Check sheet for the modelled part. Datum: model origin and axes. Units: mm. Face numbers are marked on the shaded views. A direction names the side the tool comes from. Coordinates: 2 decimals unless noted, no trailing zeros. Write each loop counter-clockwise with the first axis right and the second up, starting at its lowest first coordinate (ties: lowest second). Pieces come first, ordered by that corner, then holes. Notation, with made-up numbers: (5, 30.25) -> (10, 30.25) arc R16 cw to (10, 50.25) -> close; hole circle Ø1 at (13, 85.5). An arc over 180 degrees is marked (long way). One line per item, written item: value. Start each with the question number.
1) Gauge pin test, flat ends, axial feed: P1, Ø4, axis at x = 3, z = -9, coming from the +Y side; P2, Ø1.5, axis at y = 4, z = -2, coming from the -X side; P3, Ø1.3, axis at x = -1, y = 4, coming from the +Z side; P4, Ø0.8, axis at x = 4.5, z = -14.5, coming from the +Y side. Record the tip position at first contact, or that the pin passes through.
2) Sectioned sample at C-C on y = 1.05. Give the number of separate pieces and of enclosed holes in the cut face, plus the area to 3 significant figures.
3) Sectioned sample at A-A on z = 0. Enter the section's corners in (x, y).
4) Sectioned sample at B-B on x = 15. Enter the section's corners in (y, z).
5) Set-up check for the marked faces 4, 5 and 6: record each of +Z, -Z, +X, -X, +Y, -Y from which the full face is reachable in a straight line by a thin tool's end or side.
6) Sectioned sample at D-D on z = -6. Enter the section's corners in (x, y), plus the area to 3 significant figures.
7) Draft check along X on the marked faces 1, 2 and 3. Enter one of: +X half, -X half, draft (parallel to the pull), parting line (faces both ways), or undercut.
8) Scan lines: line 1 along Z through (x, y) = (10, 3.4); line 2 along Y through (x, z) = (14.5, 7); line 3 along Z through (x, y) = (15.5, 0.3). Record each from-to range of solid material in increasing order. Write a range as [from, to].
```python
from build123d import *

# Parameters (mm, degrees)
SKETCH1_R           = 17.5
BOSS_EXTRUDE1_DEPTH = 0.5
SKETCH2_R           = 11.5
CUT_EXTRUDE1_DEPTH  = 0.5
SKETCH3_W           = 15
SKETCH3_H           = 8
CUT_EXTRUDE4_DEPTH  = 2.5
BOSS_EXTRUDE6_DEPTH = 4.5
BOSS_EXTRUDE7_START = 4
SKETCH9_R           = 12.2
SKETCH9_R_2         = 11.5
BOSS_EXTRUDE7_DEPTH = 4
SKETCH10_W          = 4.218070674
SKETCH10_H          = 8
CUT_EXTRUDE5_DEPTH  = 6
SKETCH11_R          = 1
SKETCH11_R_2        = 0.998714777
SKETCH11_R_3        = 0.998671431
SKETCH11_R_4        = 1.032567444
SKETCH11_R_5        = 1.008118798
CUT_EXTRUDE7_DEPTH  = 100


with BuildPart() as part:
    # Sketch1 → Boss-Extrude1 (new body)
    with BuildSketch(Plane(origin=(0, 0, 0), x_dir=(1, 0, 0), z_dir=(0, 1, 0))):
        with Locations(Location((0, 0, 0), (0, 0, 270))):
            Circle(SKETCH1_R)
    extrude(amount=BOSS_EXTRUDE1_DEPTH)

    # Sketch2 → Cut-Extrude1 (cut)
    with BuildSketch(Plane(origin=(0, 0.5, 0), x_dir=(1, 0, 0), z_dir=(0, 1, 0))):
        with Locations(Location((2, 0, 0), (0, 0, 270))):
            Circle(SKETCH2_R)
    extrude(amount=-CUT_EXTRUDE1_DEPTH, mode=Mode.SUBTRACT)

    # Sketch3 → Cut-Extrude4 (cut)
    with BuildSketch(Plane(origin=(0, 0, 0), x_dir=(1, 0, 0), z_dir=(0, 1, 0))):
        with Locations((-5.5, 0)):
            Rectangle(SKETCH3_W, SKETCH3_H)
    extrude(amount=CUT_EXTRUDE4_DEPTH, mode=Mode.SUBTRACT)

    # Sketch7 → Boss-Extrude6 (add)
    with BuildSketch(Plane(origin=(0, 0.5, 0), x_dir=(1, 0, 0), z_dir=(0, 1, 0))):
        with BuildLine():
            Line((-11.135528726, 13.5), (11.135528726, 13.5))
            ThreePointArc((11.135528726, 13.5), (10.820652744, 13.753671299), (10.5, 14))
            Line((10.5, 14), (-10.5, 14))
            ThreePointArc((-10.5, 14), (-10.820652744, 13.753671299), (-11.135528726, 13.5))
        make_face()
        with BuildLine():
            Line((12.176537068, 12.5), (-12.176537068, 12.5))
            ThreePointArc((-12.176537068, 12.5), (-12.42556977, 12.252480192), (-12.669572012, 12))
            Line((-12.669572012, 12), (12.669572012, 12))
            ThreePointArc((12.669572012, 12), (12.42556977, 12.252480192), (12.176537068, 12.5))
        make_face()
        with BuildLine():
            ThreePointArc((-11.145229996, -13.491992008), (-10.830835088, -13.74565427), (-10.510668849, -13.991992008))
            Line((-10.510668849, -13.991992008), (10.510668849, -13.991992008))
            ThreePointArc((10.510668849, -13.991992008), (10.53333572, -13.974936086), (10.555974914, -13.957843444))
            Line((10.555974914, -13.957843444), (10.555974914, -13.491992008))
            Line((10.555974914, -13.491992008), (-11.145229996, -13.491992008))
        make_face()
        with BuildLine():
            Line((-9.013878189, 15), (9.013878189, 15))
            ThreePointArc((9.013878189, 15), (8.572604405, 15.256488905), (8.124038405, 15.5))
            Line((8.124038405, 15.5), (-8.124038405, 15.5))
            ThreePointArc((-8.124038405, 15.5), (-8.572604405, 15.256488905), (-9.013878189, 15))
        make_face()
        with BuildLine():
            ThreePointArc((-9.027190906, -14.991992008), (-8.586884855, -15.248455938), (-8.139298719, -15.491992008))
            Line((-8.139298719, -15.491992008), (8.139298719, -15.491992008))
            ThreePointArc((8.139298719, -15.491992008), (8.586884855, -15.248455938), (9.027190906, -14.991992008))
            Line((9.027190906, -14.991992008), (-9.027190906, -14.991992008))
        make_face()
        with BuildLine():
            Line((-5.830951895, 16.5), (5.830951895, 16.5))
            ThreePointArc((5.830951895, 16.5), (4.998387844, 16.770990399), (4.153311931, 17))
            Line((4.153311931, 17), (-4.153311931, 17))
            ThreePointArc((-4.153311931, 17), (-4.998387844, 16.770990399), (-5.830951895, 16.5))
        make_face()
        with BuildLine():
            Line((5.853562985, -16.491992008), (-5.853562985, -16.491992008))
            ThreePointArc((-5.853562985, -16.491992008), (-5.025979841, -16.762742217), (-4.185953609, -16.991992008))
            Line((-4.185953609, -16.991992008), (4.185953609, -16.991992008))
            ThreePointArc((4.185953609, -16.991992008), (5.025979841, -16.762742217), (5.853562985, -16.491992008))
        make_face()
        with BuildLine():
            Line((12.669572012, -12), (-12.669572012, -12))
            ThreePointArc((-12.669572012, -12), (-12.42556977, -12.252480192), (-12.176537068, -12.5))
            Line((-12.176537068, -12.5), (12.176537068, -12.5))
            ThreePointArc((12.176537068, -12.5), (12.42556977, -12.252480192), (12.669572012, -12))
        make_face()
    extrude(amount=BOSS_EXTRUDE6_DEPTH)

    # Sketch9 → Boss-Extrude7 (add)
    with BuildSketch(Plane(origin=(0, 0.5, 0), x_dir=(1, 0, 0), z_dir=(0, 1, 0)).offset(BOSS_EXTRUDE7_START)):
        with Locations((2, 0)):
            Circle(SKETCH9_R)
        with Locations(Location((2, 0, 0), (0, 0, 270))):
            Circle(SKETCH9_R_2, mode=Mode.SUBTRACT)
    extrude(amount=-BOSS_EXTRUDE7_DEPTH)

    # Sketch10 → Cut-Extrude5 (cut)
    with BuildSketch(Plane.XZ):
        with Locations((-10.890964663, 0)):
            Rectangle(SKETCH10_W, SKETCH10_H)
    extrude(amount=-CUT_EXTRUDE5_DEPTH, mode=Mode.SUBTRACT)

    # Sketch11 → Cut-Extrude7 (cut)
    with BuildSketch(Plane.XZ):
        with Locations(Location((-7.340296828, -10.142549821, 0), (0, 0, 270))):
            Circle(SKETCH11_R)
        with Locations((-1.767569388, -10.865331146)):
            Circle(SKETCH11_R_2)
        with Locations((5.429630438, -10.976685978)):
            Circle(SKETCH11_R_3)
        with Locations(Location((-7.340296828, 9.917402438, 0), (0, 0, 270))):
            Circle(SKETCH11_R)
        with Locations((5.429630438, 10.976685978)):
            Circle(SKETCH11_R_4)
        with Locations((-1.767569388, 10.976685978)):
            Circle(SKETCH11_R)
        with Locations(Location((10.013638897, 10.643798729, 0), (0, 0, 270))):
            Circle(SKETCH11_R_5)
        with Locations(Location((9.772353005, -10.712194768, 0), (0, 0, 270))):
            Circle(SKETCH11_R)
    extrude(amount=-CUT_EXTRUDE7_DEPTH, mode=Mode.SUBTRACT)


solid = part.part
```
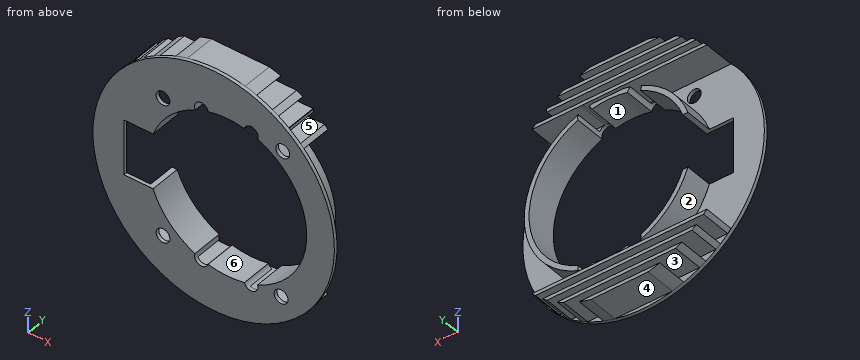
Answers:
1. P1: passes through
1. P2: stops at x = 13.17
1. P3: stops at z = 16.99
1. P4: stops at y = 0.5
2. separate pieces: 11
2. enclosed holes: 0
2. area: 114 mm2
3. outline: (-17.5, 0) -> (-13, 0) -> (-13, 0.5) -> (-17.5, 0.5) -> close; (13.5, 0) -> (17.5, 0) -> (17.5, 0.5) -> (14.2, 0.5) -> (14.2, 4.5) -> (13.5, 4.5) -> close
4. outline: (0, -9.01) -> (0.5, -9.01) -> (0.5, 9.01) -> (0, 9.01) -> close
5. face 4: -Z, +X, -X, +Y
5. face 5: +X, -X, +Y
5. face 6: +Y, -Y
6. outline: (-16.44, 0) -> (-7.81, 0) -> (-7.81, 4.5) -> (-8.62, 4.5) -> (-8.62, 0.5) -> (-16.44, 0.5) -> close; (11.81, 0) -> (16.44, 0) -> (16.44, 0.5) -> (12.62, 0.5) -> (12.62, 4.5) -> (11.81, 4.5) -> close
6. area: 13.1 mm2
7. face 1: undercut
7. face 2: -X half
7. face 3: draft
8. line 1: z = [-14, -13.5], [-12.5, -12], [-9.21, -8.26], [8.26, 9.21], [12, 12.5], [13.49, 13.99]
8. line 2: y = [0, 0.5]
8. line 3: z = [-8.12, 8.12]
